from build123d import *

# Parameters (mm, degrees)
SKETCH_R        = 37.5
PAD_DEPTH       = 5
SKETCH001_W     = 10
SKETCH001_H     = 6
SKETCH001_W_2   = 6
SKETCH001_H_2   = 10
PAD001_DEPTH    = 10
POCKET_DEPTH    = 3
POCKET001_DEPTH = 3
POCKET002_DEPTH = 3
POCKET003_DEPTH = 3
SKETCH006_R     = 2.25
POCKET004_DEPTH = 75
SKETCH007_R     = 2.25
POCKET005_DEPTH = 75
SKETCH008_R     = 2.65
POCKET006_DEPTH = 5
SKETCH009_W     = 3.74627
SKETCH009_H     = 0.45
PAD002_DEPTH    = 5
SKETCH010_R     = 40
SKETCH010_R_2   = 37.5
POCKET007_DEPTH = 15
FILLET_R        = 2
SKETCH011_R     = 3.951065
PAD003_DEPTH    = 3
FILLET001_R     = 2


with BuildPart() as part:
    # Sketch → Pad (new body)
    with BuildSketch(Plane.XY):
        Circle(SKETCH_R)
    extrude(amount=PAD_DEPTH)

    # Sketch001 (on Face3 of Pad) → Pad001 (join)
    with BuildSketch(Plane.XY.offset(5)):
        with Locations((0, 34.5)):
            Rectangle(SKETCH001_W, SKETCH001_H)
        with Locations((0, -34.5)):
            Rectangle(SKETCH001_W, SKETCH001_H)
        with Locations((-34.5, 0)):
            Rectangle(SKETCH001_W_2, SKETCH001_H_2)
        with Locations((34.5, 0)):
            Rectangle(SKETCH001_W_2, SKETCH001_H_2)
    extrude(amount=PAD001_DEPTH)

    # Sketch002 (on Face20 of Pad001) → Pocket (cut)
    with BuildSketch(Plane.YZ.offset(-31.5)):
        Polygon((4.041452, 10), (2.020726, 13.5), (-2.020726, 13.5), (-4.041452, 10), (-2.020726, 6.5), (2.020726, 6.5), align=None)
    extrude(amount=-POCKET_DEPTH, mode=Mode.SUBTRACT)

    # Sketch003 (on Face23 of Pocket) → Pocket001 (cut)
    with BuildSketch(Plane.XZ.offset(-31.5)):
        Polygon((4.041452, 10), (2.020726, 13.5), (-2.020726, 13.5), (-4.041452, 10), (-2.020726, 6.5), (2.020726, 6.5), align=None)
    extrude(amount=-POCKET001_DEPTH, mode=Mode.SUBTRACT)

    # Sketch004 (on Face15 of Pocket001) → Pocket002 (cut)
    with BuildSketch(Plane(origin=(31.5, 0, 0), x_dir=(0, -1, 0), z_dir=(-1, 0, 0))):
        Polygon((4.041452, 10), (2.020726, 13.5), (-2.020726, 13.5), (-4.041452, 10), (-2.020726, 6.5), (2.020726, 6.5), align=None)
    extrude(amount=-POCKET002_DEPTH, mode=Mode.SUBTRACT)

    # Sketch005 (on Face17 of Pocket002) → Pocket003 (cut)
    with BuildSketch(Plane(origin=(0, -31.5, 0), x_dir=(-1, 0, 0), z_dir=(0, 1, 0))):
        Polygon((4.041452, 10), (2.020726, 13.5), (-2.020726, 13.5), (-4.041452, 10), (-2.020726, 6.5), (2.020726, 6.5), align=None)
    extrude(amount=-POCKET003_DEPTH, mode=Mode.SUBTRACT)

    # Sketch006 (on Face12 of Pocket003) → Pocket004 (cut)
    with BuildSketch(Plane.YZ.offset(37.5)):
        with Locations((0, 10)):
            Circle(SKETCH006_R)
    extrude(amount=-POCKET004_DEPTH, mode=Mode.SUBTRACT)

    # Sketch007 (on Face25 of Pocket004) → Pocket005 (cut)
    with BuildSketch(Plane.XZ.offset(37.5)):
        with Locations((0, 10)):
            Circle(SKETCH007_R)
    extrude(amount=-POCKET005_DEPTH, mode=Mode.SUBTRACT)

    # Sketch008 (on Face2 of Pocket005) → Pocket006 (cut)
    with BuildSketch(Plane(origin=(0, 0, 0), x_dir=(1, 0, 0), z_dir=(0, 0, -1))):
        Circle(SKETCH008_R)
    extrude(amount=-POCKET006_DEPTH, mode=Mode.SUBTRACT)

    # Sketch009 (on Face2 of Pocket006) → Pad002 (join)
    with BuildSketch(Plane(origin=(0, 0, 0), x_dir=(1, 0, 0), z_dir=(0, 0, -1))):
        with Locations((-0.090507, 2.525)):
            Rectangle(SKETCH009_W, SKETCH009_H)
    extrude(amount=-PAD002_DEPTH)

    # Sketch010 (on Face62 of Pad002) → Pocket007 (cut)
    with BuildSketch(Plane(origin=(0, 0, 0), x_dir=(1, 0, 0), z_dir=(0, 0, -1))):
        Circle(SKETCH010_R)
        Circle(SKETCH010_R_2, mode=Mode.SUBTRACT)
    extrude(amount=-POCKET007_DEPTH, mode=Mode.SUBTRACT)

    # Fillet
    fillet_edges = [part.edges().sort_by_distance(p)[0] for p in [
        (5, -34.332586, 5),
        (-5, -34.332586, 5),
        (-34.332586, -5, 5),
        (34.332586, -5, 5),
        (5, 34.332586, 5),
        (34.332586, 5, 5),
        (-34.332586, 5, 5),
        (-5, 34.332586, 5),
    ]]
    fillet(fillet_edges, radius=FILLET_R)

    # Sketch011 (on Face1 of Fillet) → Pad003 (join)
    with BuildSketch(Plane.XY.offset(5)):
        Circle(SKETCH011_R)
    extrude(amount=PAD003_DEPTH)

    # Fillet001
    fillet001_edges = [part.edges().sort_by_distance(p)[0] for p in [
        (-3.951065, 0, 8),
    ]]
    fillet(fillet001_edges, radius=FILLET001_R)


solid = part.part
Design review of the part built by this model. Coordinates are the model's own, in mm. A direction names the side the tool comes from. Round coordinates to 2 decimals unless told otherwise and drop trailing zeros. Write each loop counter-clockwise with the first axis right and the second up, starting at its lowest first coordinate (ties: lowest second). Pieces come first, ordered by that corner, then holes.
Item 1: For faces 1 (the flat face through (-1, 9, 5)), 2 (the flat face through (-2, -34.5, 12)), 3 (the flat face through (5, -34, 11)), list the 3-axis set-ups (+Z, -Z, +X, -X, +Y, -Y) from which the entire face can be reached by the end or side of a thin tool; tool diameter is ignored.
Item 2: Draft analysis for pull direction Y (two halves, no side actions). For faces 4 (the flat face through (-32.979, 3.045, 11.726)), 5 (the flat face through (-34, -5, 11)), 6 (the flat face through (-31.5, -3.2, 7.7)), state which applies: released by +Y, released by -Y, zero draft, split by the parting line, or undercut.
Item 3: Wall thickness on L1, parallel to Z at x = -35.45, y = 0; L2, parallel to Y at x = 0, z = 2.65; L3, parallel to X at y = 0, z = 3.6: over which ranges is each line inside the solid? List them lowest first.
Item 4: For pin 1 Ø3.5 at (x, z) = (0, 9) entering from +Y; pin 2 Ø4.5 at (x, z) = (-34.5, 12) entering from -Y; pin 3 Ø1.2 at (x, y) = (0, 1) entering from +Z; pin 4 Ø3 at (y, z) = (33, 11.5) entering from -X, all flat-tipped, find the tip position at first contact; note any pin that passes through.
Item 5: Consider section C-C on z = 3.75. Give the boundary of the cut face in (x, y), and give its area (3 significant figures).
Item 6: Consider section A-A on x = 0. Count the separate pieces of the cut face and the enclosed holes in it, and give its area (3 significant figures).
Item 7: Consider section D-D on x = 23.5. Give the boundary of the cut face in (y, z).
Check values:
1. face 1: +Z
1. face 2: none
1. face 3: +Z, +X, +Y, -Y
2. face 4: undercut
2. face 5: released by -Y
2. face 6: zero draft
3. L1: z = 0 to 7.75, 12.25 to 15
3. L2: y = -37.5 to -2.3, 2.65 to 37.5
3. L3: x = -37.5 to -2.65, 2.65 to 37.5
4. pin 1: stops at y = 37.5
4. pin 2: stops at y = -5
4. pin 3: stops at z = 8
4. pin 4: stops at x = -5
5. outline: circle Ø75 at (0, 0); hole (-1.32, -2.3) - (1.32, -2.3) arc R2.65 ccw (long way) to start
5. area: 4,400 mm2
6. separate pieces: 3
6. enclosed holes: 0
6. area: 423 mm2
7. outline: (-29.22, 0) - (29.22, 0) - (29.22, 5) - (-29.22, 5) - close
